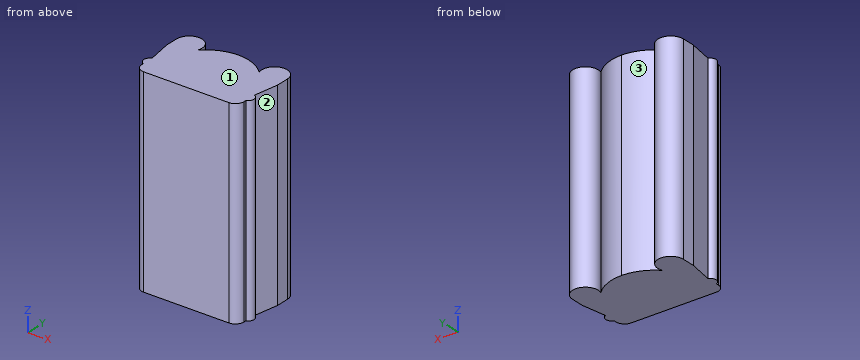
```python
from build123d import *

# Parameters (mm, degrees)
BOSS_EXTRUDE1_DEPTH = 295.656
FILLET1_R           = 12.7


with BuildPart() as part:
    # Sketch1 → Boss-Extrude1 (new body)
    with BuildSketch(Plane.XY):
        with BuildLine():
            Line((82.55, 88.9), (82.55, 69.85))
            Line((82.55, 69.85), (76.2, 33.02))
            ThreePointArc((76.2, 33.02), (82.042, 24.668844631), (76.2, 16.317689262))
            Line((76.2, 16.317689262), (76.2, 0))
            Line((76.2, 0), (-76.2, 0))
            Line((-76.2, 0), (-76.2, 16.317689262))
            ThreePointArc((-76.2, 16.317689262), (-82.042, 24.668844631), (-76.2, 33.02))
            Line((-76.2, 33.02), (-82.55, 69.85))
            Line((-82.55, 69.85), (-82.55, 88.9))
            ThreePointArc((-82.55, 88.9), (-60.192002215, 107.660587695), (-45.598855574, 82.38451627))
            ThreePointArc((-45.598855574, 82.38451627), (-24.696659186, 96.450806586), (0, 101.43451627))
            ThreePointArc((0, 101.43451627), (24.696659186, 96.450806586), (45.598855574, 82.38451627))
            ThreePointArc((45.598855574, 82.38451627), (60.192002215, 107.660587695), (82.55, 88.9))
        make_face()
    extrude(amount=BOSS_EXTRUDE1_DEPTH)

    # Fillet1
    fillet1_edges = [part.edges().sort_by_distance(p)[0] for p in [
        (76.2, 0, 147.828),
        (-76.2, 0, 147.828),
    ]]
    fillet(fillet1_edges, radius=FILLET1_R)


solid = part.part
```
Input: part model. Units: mm. Frame: model coordinates. Face numbers are marked on the shaded views. Coordinates: 2 decimals unless noted, no trailing zeros. Write each loop counter-clockwise with the first axis right and the second up, starting at its lowest first coordinate (ties: lowest second). Pieces come first, ordered by that corner, then holes.
1) Pin query (flat end, axial travel): pin 1 Ø4 at (x, z) = (-36, 92.5) entering from +Y; pin 2 Ø8 at (x, y) = (-47, 91.5) entering from -Z; pin 3 Ø1.8 at (y, z) = (13.5, 216.5) entering from -X; pin 4 Ø1.1 at (y, z) = (14, 111) entering from +X. Return the tip coordinate at first contact, or that it passes through.
2) Section A-A on y = 97. Output: boundary loops of the cut face in (x, z).
3) Mould query, pull axis X, two halves, no side actions, for the marked faces 1, 2 and 3. Classes: pulls with the +X half, pulls with the -X half, needs draft (parallel to the pull), parting line crosses it, or undercut.
4) Section C-C on x = 73. Output: boundary loops of the cut face in (y, z), and give its area (3 significant figures).
5) Section B-B on z = 80.5. Output: boundary loops of the cut face in (x, y).
6) Section D-D on y = 9. Output: boundary loops of the cut face in (x, z).
7) Material intervals for line 1 along X through (y, z) = (93, 251); line 2 along X through (y, z) = (102, 128); line 3 along X through (y, z) = (13.5, 35.5), sorted ascending.
Check result:
1. pin 1: stops at y = 91.64
1. pin 2: stops at z = 0
1. pin 3: stops at x = -76.2
1. pin 4: stops at x = 76.2
2. outline: (-80.74, 0) - (-46.26, 0) - (-46.26, 295.66) - (-80.74, 295.66) - close; (-23.34, 0) - (23.34, 0) - (23.34, 295.66) - (-23.34, 295.66) - close; (46.26, 0) - (80.74, 0) - (80.74, 295.66) - (46.26, 295.66) - close
3. face 1: needs draft
3. face 2: pulls with the +X half
3. face 3: undercut
4. outline: (4.27, 0) - (105.41, 0) - (105.41, 295.66) - (4.27, 295.66) - close
4. area: 29,900 mm2
5. outline: (-82.55, 69.85) - (-76.2, 33.02) arc R8.89 ccw to (-76.2, 16.32) - (-76.2, 12.7) arc R12.7 ccw to (-63.5, 0) - (63.5, 0) arc R12.7 ccw to (76.2, 12.7) - (76.2, 16.32) arc R8.89 ccw to (76.2, 33.02) - (82.55, 69.85) - (82.55, 88.9) arc R19.05 ccw (long way) to (45.6, 82.38) arc R64.49 ccw to (0, 101.43) arc R64.49 ccw to (-45.6, 82.38) arc R19.05 ccw (long way) to (-82.55, 88.9) - close
6. outline: (-75.65, 0) - (75.65, 0) - (75.65, 295.66) - (-75.65, 295.66) - close
7. line 1: x = -82.1 to -44.9, -31.72 to 31.72, 44.9 to 82.1
7. line 2: x = -77.33 to -49.67, 49.67 to 77.33
7. line 3: x = -76.2 to 76.2
